Can you work these out from the model? Positions are in its coordinate system, mm. Round coordinates to 2 decimals unless told otherwise and drop trailing zeros. Loops run counter-clockwise (first coordinate to the right, second up) from the corner with the lowest first, then second, coordinate; pieces in that order, holes last.
(1) I want a section at A-A on z = 0.95. Give the number of separate pieces and of enclosed holes in the cut face, plus the area to 3 significant figures.
(2) If I drill on line 1 along Y through (x, z) = (0, 1); line 2 along X through (y, z) = (3, 1.2); line 3 along X through (y, z) = (7, 0.55), over which ranges is the centre line in solid material (lowest first)?
(3) I want a section at C-C on y = 14. Write out the boundary of the cut face in (x, z), plus the area to 3 significant figures.
(4) I want a section at B-B on y = -14.5. Write out the boundary of the cut face in (x, z), plus the area to 3 significant figures.
(5) Will these pins go through, and if not, where does the flat tip stop? pin 1 Ø1.5 at (x, z) = (-31, 2) entering from +Y; pin 2 Ø17.5 at (x, y) = (0, 0) entering from -Z.
from build123d import *

# Parameters (mm, degrees)
F0_R     = 11
F1_DEPTH = 3


with BuildPart() as f1:
    # F0 (on Top) → F1 (new body)
    with BuildSketch(Plane.XY):
        with BuildLine():
            ThreePointArc((23.7810725764, 32.7823697802), (14.799332437, 45.661578591), (-0.0297016333, 40.4996580122))
            ThreePointArc((-0.0297016333, 40.4996580122), (-14.8662910452, 45.6398224203), (-23.8291308285, 32.7474534162))
            ThreePointArc((-23.8291308285, 32.7474534162), (-38.8534966348, 28.1852053257), (-38.5266419697, 12.4868346603))
            ThreePointArc((-38.5266419697, 12.4868346603), (-47.9999870917, -0.0352022235), (-38.5082853508, -12.543330524))
            ThreePointArc((-38.5082853508, -12.543330524), (-38.8121139391, -28.2421637198), (-23.7810725764, -32.7823697802))
            ThreePointArc((-23.7810725764, -32.7823697802), (-14.799332437, -45.661578591), (0.0297016333, -40.4996580122))
            ThreePointArc((0.0297016333, -40.4996580122), (14.8662910452, -45.6398224203), (23.8291308285, -32.7474534162))
            ThreePointArc((23.8291308285, -32.7474534162), (38.8534966348, -28.1852053257), (38.5266419697, -12.4868346603))
            ThreePointArc((38.5266419697, -12.4868346603), (47.9999870917, 0.0352022235), (38.5082853508, 12.543330524))
            ThreePointArc((38.5082853508, 12.543330524), (38.8121139391, 28.2421637198), (23.7810725764, 32.7823697802))
        make_face()
        Polygon((-9.4205159653, -29.0658806367), (-6.4434088175, -32.3674206355), (-7.8140727542, -36.5964410547), (-12.1618438387, -37.5239214751), (-15.1389509865, -34.2223814763), (-13.7682870498, -29.9933610571), align=None, mode=Mode.SUBTRACT)
        Polygon((-24.7058534949, -17.9775510382), (-24.2379197394, -22.3984526808), (-27.8325659918, -25.0141460217), (-31.8951459997, -23.2089377199), (-32.3630797552, -18.7880360772), (-28.7684335028, -16.1723427364), align=None, mode=Mode.SUBTRACT)
        Polygon((-30.5543947105, -0.0224079775), (-32.7743691374, -3.8740370974), (-37.2199650146, -3.8772974079), (-39.4455864649, -0.0289285984), (-37.225612038, 3.8227005214), (-32.7800161608, 3.8259608319), align=None, mode=Mode.SUBTRACT)
        Polygon((-14.445933389, -15.8846642147), (-10.7412099068, -18.3419711254), (-11.0169383754, -22.7790092304), (-14.9973903261, -24.7587404246), (-18.7021138083, -22.3014335138), (-18.4263853398, -17.8643954088), align=None, mode=Mode.SUBTRACT)
        Polygon((-21.0237769743, -4.3598566979), (-19.4709614803, -8.5254415758), (-22.3020560592, -11.95301168), (-26.685966132, -11.2149969062), (-28.2387816261, -7.0494120284), (-25.4076870472, -3.6218419242), align=None, mode=Mode.SUBTRACT)
        Polygon((9.4631384714, -29.052031745), (13.8122652692, -29.9731340357), (15.1891306849, -34.2001394722), (12.2168693028, -37.506042618), (7.867742505, -36.5849403273), (6.4908770893, -32.3579348908), align=None, mode=Mode.SUBTRACT)
        Polygon((-2.3502342483, -21.3420699013), (2.0913187707, -21.1524911258), (4.4762753158, -24.9041994849), (2.4196788418, -28.8454866194), (-2.0218741773, -29.0350653948), (-4.4068307223, -25.2833570358), align=None, mode=Mode.SUBTRACT)
        Polygon((10.6431744937, -18.6475302759), (14.1250347592, -15.8834784629), (18.2597039794, -17.5168319988), (18.912512934, -21.9142373476), (15.4306526685, -24.6782891606), (11.2959834483, -23.0449356247), align=None, mode=Mode.SUBTRACT)
        Polygon((19.5712523273, -8.8302678913), (20.7634675619, -4.5475168867), (25.0685463473, -3.4386300643), (28.1814098981, -6.6124942466), (26.9891946635, -10.8952452512), (22.6841158781, -12.0041320736), align=None, mode=Mode.SUBTRACT)
        Polygon((24.7321956523, -17.9412941689), (28.7921234848, -16.1301289835), (32.390602462, -18.7405470312), (31.9291536068, -23.1621302644), (27.8692257743, -24.9732954497), (24.2707467971, -22.362877402), align=None, mode=Mode.SUBTRACT)
        Polygon((-24.7321956523, 17.9412941689), (-28.7921234848, 16.1301289835), (-32.390602462, 18.7405470312), (-31.9291536068, 23.1621302644), (-27.8692257743, 24.9732954497), (-24.2707467971, 22.362877402), align=None, mode=Mode.SUBTRACT)
        Polygon((-19.5712523273, 8.8302678913), (-20.7634675619, 4.5475168867), (-25.0685463473, 3.4386300643), (-28.1814098981, 6.6124942466), (-26.9891946635, 10.8952452512), (-22.6841158781, 12.0041320736), align=None, mode=Mode.SUBTRACT)
        Circle(F0_R, mode=Mode.SUBTRACT)
        Polygon((-10.6431744937, 18.6475302759), (-14.1250347592, 15.8834784629), (-18.2597039794, 17.5168319988), (-18.912512934, 21.9142373476), (-18.143609215, 22.524626495), (-15.4306526685, 24.6782891606), (-11.2959834483, 23.0449356247), align=None, mode=Mode.SUBTRACT)
        Polygon((2.3502342483, 21.3420699013), (-2.0913187707, 21.1524911258), (-4.4762753158, 24.9041994849), (-2.4196788418, 28.8454866194), (2.0218741773, 29.0350653948), (4.4068307223, 25.2833570358), align=None, mode=Mode.SUBTRACT)
        Polygon((-9.4631384714, 29.052031745), (-13.8122652692, 29.9731340357), (-15.1891306849, 34.2001394722), (-12.2168693028, 37.506042618), (-7.867742505, 36.5849403273), (-6.4908770893, 32.3579348908), align=None, mode=Mode.SUBTRACT)
        Polygon((26.685966132, 11.2149969062), (28.2387816261, 7.0494120284), (25.4076870472, 3.6218419242), (21.0237769743, 4.3598566979), (19.4709614803, 8.5254415758), (22.3020560592, 11.95301168), align=None, mode=Mode.SUBTRACT)
        Polygon((14.445933389, 15.8846642147), (10.7412099068, 18.3419711254), (11.0169383754, 22.7790092304), (14.9973903261, 24.7587404246), (18.7021138083, 22.3014335138), (18.4263853398, 17.8643954088), align=None, mode=Mode.SUBTRACT)
        Polygon((39.4455864649, 0.0289285984), (37.225612038, -3.8227005214), (32.7800161608, -3.8259608319), (30.5543947105, 0.0224079775), (32.7743691374, 3.8740370974), (37.2199650146, 3.8772974079), align=None, mode=Mode.SUBTRACT)
        Polygon((24.7058534949, 17.9775510382), (24.2379197394, 22.3984526808), (27.8325659918, 25.0141460217), (31.8951459997, 23.2089377199), (32.3630797552, 18.7880360772), (28.7684335028, 16.1723427364), align=None, mode=Mode.SUBTRACT)
        Polygon((9.4205159653, 29.0658806367), (6.4434088175, 32.3674206355), (7.8140727542, 36.5964410547), (12.1618438387, 37.5239214751), (15.1389509865, 34.2223814763), (13.7682870498, 29.9933610571), align=None, mode=Mode.SUBTRACT)
    extrude(amount=F1_DEPTH)


solid = f1.part
Filled sheet:
1. separate pieces: 1
1. enclosed holes: 21
1. area: 5,160 mm2
2. line 1: y = -40.54 to -28.95, -21.24 to -11, 11 to 21.24, 28.95 to 40.54
2. line 2: x = -47.64 to -37.7, -32.3 to -10.58, 10.58 to 32.27, 37.73 to 47.66
2. line 3: x = -45.94 to -28.07, -20.08 to -8.49, 8.49 to 20.04, 28.2 to 45.97
3. outline: (-39.56, 0) - (39.5, 0) - (39.5, 3) - (-39.56, 3) - close
3. area: 237 mm2
4. outline: (-39.78, 0) - (39.84, 0) - (39.84, 3) - (-39.78, 3) - close
4. area: 239 mm2
5. pin 1: stops at y = 33.41
5. pin 2: passes through
